Read the model definition and answer for the solid it produces. Units are mm, in the model's axes. A direction names the side the tool comes from. Round coordinates to 2 decimals unless told otherwise and drop trailing zeros. Order: outer loops, then holes, each group sorted by start corner. A loop starts at its lowest first (then second) coordinate and runs counter-clockwise, first axis right, second up. Notation, with made-up numbers: (6, 6) -> (46, 6) arc R18 cw to (46, 28) -> close; hole circle Ø5 at (-37, 59.5). An arc over 180 degrees is marked (long way). Use a Markdown table: item, result. Add a question column.
1. For faces 1 (the face through (36.005, 48, 31)), 2 (the face through (176, 47, 31)), 3 (the face through (105, 0, 31)), determine the directions among +Z, -Z, +X, -X, +Y, -Y from which every point of the face is accessible in a straight line to the end or side of a thin tool.
2. Consider L1, parallel to Y at x = 185, z = 12; L2, parallel to X at y = 40, z = 23; L3, parallel to X at y = 59.5, z = 3.5 (1 decimal). Determine where each line is inside the solid, lowest interval first. Write a range as [from, to].
3. The mould has two halves that part along X. Classify faces 4 (the face through (89.24, 57.39, 31.06)), 5 (the face through (54, 69.633, 31)), 6 (the face through (211, 23, 32)), 7 (the face through (123.2, 57.7, 31.1)): +X half, -X half, draft (parallel to the pull), parting line (faces both ways), or undercut.
4. Section A-A, the plane y = 57 is taken. Give the vertices of the cut face in (x, z).
5. Section C-C, the plane x = 26.5 is taken. Give the vertices of the cut face in (y, z), then the cut area to 4 significant figures.
6. Section D-D, the plane x = 133.5 is taken. Give the vertices of the cut face in (y, z).
7. Given pin 1 (22.5 mm diameter, centred on y = 37.5, z = 39.5, fed in from -X); pin 2 (22.5 mm diameter, centred on y = 37.5, z = 40.5, fed in from +X); pin 3 (25 mm diameter, centred on x = 20.5, z = 21, fed in from +Y), each flat-ended and moving along its own axis, determine where each tip first touches the part or whether it passes through.
8. Section B-B, the plane z = 7 is taken. Give the vertices of the cut face in (x, y), then the cut area to 3 significant figures.
```python
from build123d import *

# Parameters (mm, degrees)
BOSS_EXTRUDE1_DEPTH = 63
FILLET1_R           = 5
FILLET2_R           = 5


with BuildPart() as part:
    # Sketch1 → Boss-Extrude1 (new body)
    with BuildSketch(Plane.XY):
        Polygon((0, 0), (212, 0), (212, 25), (176, 25), (176, 69.632533644), (140, 69.632533644), (106.004578334, 45.485327779), (72.004578334, 69.632533644), (36.004578334, 69.632533644), (36.004578334, 25), (0, 25), align=None)
    extrude(amount=BOSS_EXTRUDE1_DEPTH)

    # Fillet1
    fillet1_edges = [part.edges().sort_by_distance(p)[0] for p in [
        (212, 25, 31.5),
    ]]
    fillet(fillet1_edges, radius=FILLET1_R)

    # Fillet2
    fillet2_edges = [part.edges().sort_by_distance(p)[0] for p in [
        (0, 25, 31.5),
    ]]
    fillet(fillet2_edges, radius=FILLET2_R)


solid = part.part
```
Verdict:
| question | item | result |
|---|---|---|
| 1 | face 1 | +Z, -Z, -X, +Y |
| 1 | face 2 | +Z, -Z, +X, +Y |
| 1 | face 3 | +Z, -Z, +X, -X, -Y |
| 2 | L1 | y = [0, 25] |
| 2 | L2 | x = [36, 176] |
| 2 | L3 | x = [36, 86.3], [125.7, 176] |
| 3 | face 4 | undercut |
| 3 | face 5 | draft |
| 3 | face 6 | +X half |
| 3 | face 7 | undercut |
| 4 | outline | (36, 0) -> (89.79, 0) -> (89.79, 63) -> (36, 63) -> close; (122.22, 0) -> (176, 0) -> (176, 63) -> (122.22, 63) -> close |
| 5 | outline | (0, 0) -> (25, 0) -> (25, 63) -> (0, 63) -> close |
| 5 | area | 1,575 mm2 |
| 6 | outline | (0, 0) -> (65.02, 0) -> (65.02, 63) -> (0, 63) -> close |
| 7 | pin 1 | stops at x = 36 |
| 7 | pin 2 | stops at x = 176 |
| 7 | pin 3 | stops at y = 25 |
| 8 | outline | (0, 0) -> (212, 0) -> (212, 20) arc R5 ccw to (207, 25) -> (176, 25) -> (176, 69.63) -> (140, 69.63) -> (106, 45.49) -> (72, 69.63) -> (36, 69.63) -> (36, 25) -> (5, 25) arc R5 ccw to (0, 20) -> close |
| 8 | area | 10,700 mm2 |
